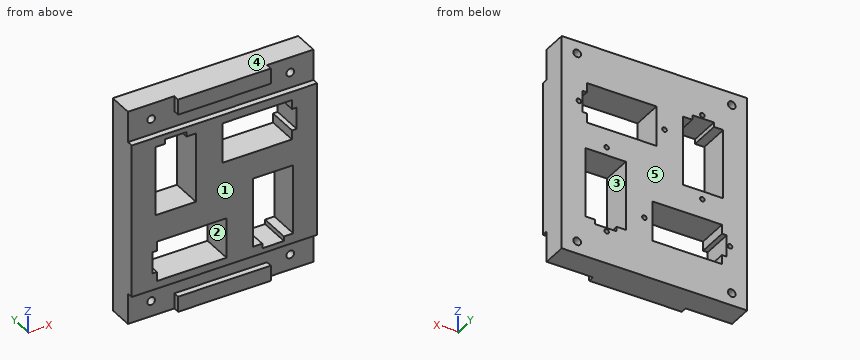
Autodesk Inventor part; units mm, degrees
ref_plane "YZ Plane" through (0, 0, 0) normal (1, 0, 0) x (0, 1, 0)
ref_plane "XZ Plane" through (0, 0, 0) normal (0, 1, 0) x (-1, 0, 0)
ref_plane "XY Plane" through (0, 0, 0) normal (0, 0, 1) x (1, 0, 0)
sketch "Skizze1" plane through (0, 0, 0) normal (0, 1, 0) x (-1, 0, 0)
  line L0 (30, -35) -> (-30, -35)
  line L1 (-30, -35) -> (-30, 35)
  line L2 (-30, 35) -> (30, 35)
  line L3 (30, 35) -> (30, -35)
  line L4 (30, -35) -> (-30, 35) construction
  line L5 (-30, -35) -> (30, 35) construction
  point P0 (0, 0)
  dimension "d0" = 60
  dimension "d1" = 70
extrude "Extrusion1" add sketch "Skizze1" along normal blind 10
sketch "Skizze2" plane through (0, 10, 0) normal (0, 1, 0) x (1, 0, 0)
  circle A0 centre (-15.75, 15.75) radius 1.75
  circle A1 centre (15.75, 15.75) radius 1.75
  circle A2 centre (15.75, -15.75) radius 1.75
  circle A3 centre (-15.75, -15.75) radius 1.75
  line L0 (42, 0) -> (-42, 0)
  line L1 (0, 49) -> (0, -49)
  point P0 (0, 0)
  dimension "d4" = 31.5
  dimension "d5" = 31.5
  dimension "d6" = 15.75
  dimension "d7" = 31.5
  dimension "d8" = 31.5
  dimension "d9" = 15.75
  dimension "d10" = 15.75
  dimension "d11" = 15.75
  dimension "d12" = 3.5
  dimension "d13" = 3.5
  dimension "d14" = 3.5
  dimension "d15" = 3.5
extrude "Extrusion2" cut sketch "Skizze2" against normal blind 10
sketch "Skizze3" plane through (0, 10, 0) normal (0, 1, 0) x (1, 0, 0)
  circle A0 centre (-15.75, 15.75) radius 1.75
  circle A1 centre (-15.75, 15.75) radius 5
  circle A2 centre (15.75, 15.75) radius 1.75
  circle A3 centre (15.75, 15.75) radius 5
  circle A4 centre (15.75, -15.75) radius 1.75
  circle A5 centre (15.75, -15.75) radius 5
  circle A6 centre (-15.75, -15.75) radius 1.75
  circle A7 centre (-15.75, -15.75) radius 5
  point P0 (0, 0)
  dimension "d18" = 10
  dimension "d19" = 10
  dimension "d20" = 10
  dimension "d21" = 10
extrude "Extrusion3" cut sketch "Skizze3" against normal blind 7 contours A0 | A1 | A2 | A3 | A4 | A5 | A6 | A7
sketch "Skizze6" plane through (0, 0, 0) normal (0, 1, 0) x (-1, 0, 0)
  line L0 (37.5, 25) -> (-37.5, 25)
  line L1 (37.5, -25) -> (-37.5, -25)
  line L2 (37.5, 40) -> (15, 40)
  line L3 (15, 40) -> (15, 30)
  line L4 (-37.5, 40) -> (-15, 40)
  line L5 (-15, 40) -> (-15, 30)
  line L6 (0, -45.47) -> (0, 45.495)
  line L7 (37.5, -40) -> (15, -40)
  line L8 (15, -40) -> (15, -30)
  line L9 (-37.5, -40) -> (-15, -40)
  line L10 (-15, -40) -> (-15, -30)
  line L11 (-15, 30) -> (15, 30)
  line L12 (-15, -30) -> (15, -30)
  line L13 (-37.5, 25) -> (-37.5, 40)
  line L14 (37.5, 40) -> (37.5, 25)
  line L15 (-37.5, -25) -> (-37.5, -40)
  line L16 (-30, 35) -> (-30, -35)
  line L17 (37.5, -25) -> (37.5, -40)
  point P0 (0, 0)
  dimension "d37" = 10
  dimension "d38" = 15
  dimension "d39" = 15
  dimension "d40" = 75
  dimension "d43" = 10
  dimension "d44" = 15
  dimension "d45" = 15
  dimension "d46" = 22.5
  dimension "d47" = 22.5
  dimension "d48" = 22.5
  dimension "d49" = 75
  dimension "d50" = 22.5
  dimension "d76" = 5
  dimension "d77" = 25
  dimension "d78" = 5
  dimension "d79" = 25
extrude "Extrusion6" cut sketch "Skizze6" along normal blind 2 contours L0 L6 L11 L3 L2 L14 | L0 L13 L4 L5 L11 L6 | L6 L12 L10 L9 L15 L1 | L1 L17 L7 L8 L12 L6
sketch "Skizze7" plane through (0, 2, 0) normal (0, -1, 0) x (1, 0, 0)
  circle A0 centre (-22.5, 30) radius 1.25
  circle A1 centre (22.5, 30) radius 1.25
  circle A2 centre (22.5, -30) radius 1.25
  circle A3 centre (-22.5, -30) radius 1.25
  line L0 (0, 49) -> (0, -49)
  line L1 (-42, 0) -> (42, 0)
  point P0 (0, 0)
  dimension "d55" = 45
  dimension "d56" = 22.5
  dimension "d57" = 60
  dimension "d58" = 45
  dimension "d59" = 60
  dimension "d60" = 30
  dimension "d61" = 30
  dimension "d62" = 2.5
  dimension "d63" = 2.5
  dimension "d64" = 2.5
  dimension "d65" = 2.5
  dimension "d71" = 22.5
extrude "Extrusion7" cut sketch "Skizze7" against normal blind 6
sketch "Skizze9" plane through (0, 10, 0) normal (0, 1, 0) x (1, 0, 0)
  line L0 (-9.25, -21.85) -> (-22.25, -21.85)
  line L1 (-22.25, -21.85) -> (-22.25, 0.65)
  line L2 (-22.25, 0.65) -> (-9.25, 0.65)
  line L3 (-9.25, 0.65) -> (-9.25, -21.85)
  circle A0 centre (-15.75, -15.75) radius 1.75
  line L4 (21.85, -22.25) -> (-0.65, -22.25)
  line L5 (-0.65, -22.25) -> (-0.65, -9.25)
  line L6 (-0.65, -9.25) -> (21.85, -9.25)
  line L7 (21.85, -9.25) -> (21.85, -22.25)
  line L8 (22.25, 21.85) -> (9.25, 21.85)
  line L9 (9.25, 21.85) -> (9.25, -0.65)
  line L10 (9.25, -0.65) -> (22.25, -0.65)
  line L11 (22.25, -0.65) -> (22.25, 21.85)
  circle A1 centre (15.75, 15.75) radius 1.75
  line L12 (-21.85, 9.5) -> (0.65, 9.5)
  line L13 (0.65, 9.5) -> (0.65, 22.5)
  line L14 (0.65, 22.5) -> (-21.85, 22.5)
  line L15 (-21.85, 22.5) -> (-21.85, 9.5)
  circle A2 centre (15.75, -15.75) radius 1.75
  point P0 (0, 0)
  point P1 (-15.75, 16)
  dimension "d80" = 13
  dimension "d81" = 22.5
  dimension "d82" = 6.5
  dimension "d83" = 6.1
  dimension "d97" = 13
  dimension "d99" = 22.5
  dimension "d101" = 13
  dimension "d102" = 6.5
  dimension "d103" = 6.1
  dimension "d104" = 22.5
  dimension "d105" = 13
  dimension "d106" = 22.5
  dimension "d107" = 6.1
  dimension "d108" = 6.5
  dimension "d164" = 6.5
extrude "Extrusion9" cut sketch "Skizze9" against normal blind 10 contours L0 L1 L2 L3 | L4 L5 L6 L7 | L11 L10 L9 L8 | A1 | L15 L14 L13 L12 | A2
sketch "Skizze10" plane through (0, 10, 0) normal (0, 1, 0) x (1, 0, 0)
  circle A0 centre (-3.25, -15.5) radius 0.75
  circle A1 centre (24.45, -15.5) radius 0.75
  circle A2 centre (15.5, -3.25) radius 0.75
  circle A3 centre (15.5, 24.45) radius 0.75
  circle A4 centre (3.25, 15.75) radius 0.75
  circle A5 centre (-24.45, 15.75) radius 0.75
  circle A6 centre (-15.5, 3.25) radius 0.75
  circle A7 centre (-15.5, -24.45) radius 0.75
  line L0 (-22.25, 0.65) -> (-9.25, 0.65)
  line L1 (-9.25, -21.85) -> (-22.25, -21.85)
  line L2 (-21.85, 9.5) -> (-21.85, 22.5)
  line L3 (0.65, 22.5) -> (0.65, 9.5)
  line L4 (9.25, 21.85) -> (22.25, 21.85)
  line L5 (22.25, -0.65) -> (9.25, -0.65)
  line L6 (21.85, -9.25) -> (21.85, -22.25)
  line L7 (-0.65, -22.25) -> (-0.65, -9.25)
  line L8 (-9.25, 0.65) -> (-9.25, -21.85)
  line L9 (-0.65, -9.25) -> (21.85, -9.25)
  line L10 (9.25, -0.65) -> (9.25, 21.85)
  line L11 (0.65, 9.5) -> (-21.85, 9.5)
  point P0 (0, 0)
  dimension "d109" = 1.5
  dimension "d110" = 1.5
  dimension "d111" = 1.5
  dimension "d112" = 1.5
  dimension "d113" = 1.5
  dimension "d114" = 1.5
  dimension "d115" = 1.5
  dimension "d116" = 1.5
  dimension "d117" = 2.6
  dimension "d118" = 2.6
  dimension "d119" = 2.6
  dimension "d120" = 2.6
  dimension "d121" = 2.6
  dimension "d122" = 2.6
  dimension "d123" = 2.6
  dimension "d124" = 2.6
  dimension "d125" = 6.25
  dimension "d126" = 6.25
  dimension "d127" = 6.25
  dimension "d128" = 6.25
  dimension "d130" = 6.25
  dimension "d131" = 6.25
  dimension "d132" = 6.25
  dimension "d133" = 6.25
extrude "Extrusion10" cut sketch "Skizze10" against normal blind 5
sketch "Skizze11" plane through (0, 10, 0) normal (0, 1, 0) x (1, 0, 0)
  circle A0 centre (25, -31) radius 1.25
  circle A1 centre (-25, -31) radius 1.25
  circle A2 centre (-25, 31) radius 1.25
  circle A3 centre (25, 31) radius 1.25
  line L0 (-30, -35) -> (30, -35)
  line L1 (30, -35) -> (30, 35)
  point P0 (0, 0)
  dimension "d136" = 50
  dimension "d137" = 62
  dimension "d138" = 50
  dimension "d139" = 62
  dimension "d140" = 4
  dimension "d141" = 5
  dimension "d142" = 5
  dimension "d143" = 4
  dimension "d144" = 2.5
  dimension "d145" = 2.5
  dimension "d146" = 2.5
  dimension "d147" = 2.5
extrude "Extrusion11" cut sketch "Skizze11" against normal blind 5
sketch "Skizze12" plane through (0, 10, 0) normal (0, 1, 0) x (1, 0, 0)
  line L0 (-21.85, 22.5) -> (-21.85, 9.5)
  line L1 (-21.85, 12.5) -> (-23.35, 12.5)
  line L2 (-23.35, 12.5) -> (-23.35, 19.5)
  line L3 (-23.35, 19.5) -> (-21.85, 19.5)
  line L4 (-21.85, 19.5) -> (-21.85, 12.5)
  line L5 (9.25, 21.85) -> (22.25, 21.85)
  line L6 (19.25, 21.85) -> (12.25, 21.85)
  line L7 (12.25, 21.85) -> (12.25, 23.35)
  line L8 (12.25, 23.35) -> (19.25, 23.35)
  line L9 (19.25, 23.35) -> (19.25, 21.85)
  line L10 (21.85, -9.25) -> (21.85, -22.25)
  line L11 (21.85, -19.25) -> (23.35, -19.25)
  line L12 (23.35, -19.25) -> (23.35, -12.25)
  line L13 (23.35, -12.25) -> (21.85, -12.25)
  line L14 (21.85, -12.25) -> (21.85, -19.25)
  line L15 (-9.25, -21.85) -> (-22.25, -21.85)
  line L16 (-12.25, -21.85) -> (-19.25, -21.85)
  line L17 (-19.25, -21.85) -> (-19.25, -23.35)
  line L18 (-19.25, -23.35) -> (-12.25, -23.35)
  line L19 (-12.25, -23.35) -> (-12.25, -21.85)
  line L20 (21.85, -22.25) -> (-0.65, -22.25)
  line L21 (-0.65, -9.25) -> (21.85, -9.25)
  line L22 (-9.25, 0.65) -> (-9.25, -21.85)
  line L23 (-22.25, -21.85) -> (-22.25, 0.65)
  line L24 (-21.85, 22.5) -> (0.65, 22.5)
  line L25 (0.65, 9.5) -> (-21.85, 9.5)
  line L26 (9.25, -0.65) -> (9.25, 21.85)
  line L27 (22.25, 21.85) -> (22.25, -0.65)
  point P0 (0, 0)
  point P1 (-21.85, 19.5)
  dimension "d150" = 3
  dimension "d151" = 3
  dimension "d152" = 1.5
  dimension "d153" = 3
  dimension "d154" = 3
  dimension "d155" = 1.5
  dimension "d156" = 3
  dimension "d157" = 3
  dimension "d158" = 1.5
  dimension "d159" = 3
  dimension "d160" = 3
  dimension "d161" = 1.5
extrude "Extrusion12" cut sketch "Skizze12" against normal blind 10
equation "\"d6\" = 0.5 * d5"
equation "\"d9\" = 0.5 * d7"
equation "\"d10\" = 0.5 * d8"
equation "\"d11\" = 0.5 * d5"
equation "\"d56\" = 0.5 * d55"
equation "\"d60\" = 0.5 * d57"
equation "\"d61\" = 0.5 * d59"
equation "\"d71\" = 0.5 * d58"
equation "\"d82\" = 0.5 * d80"
equation "\"d102\" = 0.5 * d101"
equation "\"d164\" = 0.5 * d97"
properties part number "Fuehrungsgrundplatte_V2"
CAD build for the part. Positions are in the model's coordinates, mm. Face numbers are marked on the shaded views. A direction names the side the tool comes from. Coordinates: 2 decimals unless noted, no trailing zeros. Write each loop counter-clockwise with the first axis right and the second up, starting at its lowest first coordinate (ties: lowest second). Pieces come first, ordered by that corner, then holes. Notation, with made-up numbers: (-17.5, 16) -> (-7.5, 16) arc R24 cw to (-7.5, 51) -> close; hole circle Ø11 at (62, 14.25). An arc over 180 degrees is marked (long way). Use CSV: the item, a comma, the result in double quotes. Start each with the question number.
Item 1: Band-saw the part on D-D, the plane z = -7. Write the cut outline in (x, y).
Item 2: Wall check: probe 1 along X at (y, z) = (6.9, 15.5); probe 2 along Z at (x, y) = (15.5, 7.4); probe 3 along Z at (x, y) = (-11, 3.5). Give the ranges that are in metal, low to high.
Item 3: Band-saw the part on C-C, the plane y = 1.25. Give the number of separate pieces and of enclosed holes in the cut face, plus the area to 3 significant figures.
Item 4: Drop flat-ended pins along their axis: P1, Ø2, axis at x = 25, z = 31, coming from the +Y side; P2, Ø0.9, axis at x = 15.5, z = -24.45, coming from the -Y side; P3, Ø4, axis at x = -25, z = 31, coming from the -Y side; P4, Ø1, axis at y = 1, z = -32.5, coming from the +X side. Give the stop position or say it passes through.
Item 5: Band-saw the part on B-B, the plane x = -6. Write the cut outline in (y, z).
Item 6: Band-saw the part on A-A, the plane x = -20. Write the cut outline in (y, z).
Item 7: Tool access for the marked faces 1 and 2: list every direction of +Z, -Z, +X, -X, +Y, -Y with a clear straight run to the whole face (end or side of a thin tool).
Item 8: Two-plate mould, pull along Z, no slides. Class the marked faces 3, 4 and 5: +Z half, -Z half, draft (parallel to the pull), parting line (faces both ways), or undercut.
Response values:
1,outline,"(-30, 0) -> (9.25, 0) -> (9.25, 10) -> (-30, 10) -> close; (22.25, 0) -> (30, 0) -> (30, 10) -> (22.25, 10) -> close"
2,probe 1,"x = -30 to -22.25, -9.25 to -4, -2.5 to -0.65, 23.35 to 23.7, 25.2 to 30"
2,probe 2,"z = -35 to -25.2, -23.7 to -23.35, 0.65 to 2.5, 4 to 9.25, 22.25 to 35"
2,probe 3,"z = -35 to -22.5, -9.5 to -0.65, 21.85 to 35"
3,separate pieces,"3"
3,enclosed holes,"4"
3,area,"2,090 mm2"
4,P1,"stops at y = 5"
4,P2,"stops at y = 0"
4,P3,"stops at y = 2"
4,P4,"stops at x = 15"
5,outline,"(0, -35) -> (10, -35) -> (10, -22.5) -> (0, -22.5) -> (0, -25) -> (2, -25) -> (2, -30) -> (0, -30) -> close; (0, -9.5) -> (10, -9.5) -> (10, 35) -> (0, 35) -> (0, 30) -> (2, 30) -> (2, 25) -> (0, 25) -> close"
6,outline,"(0, -25) -> (2, -25) -> (2, -35) -> (10, -35) -> (10, -22.5) -> (0, -22.5) -> close; (0, -9.5) -> (10, -9.5) -> (10, -0.65) -> (0, -0.65) -> close; (0, 21.85) -> (10, 21.85) -> (10, 35) -> (2, 35) -> (2, 25) -> (0, 25) -> close"
7,face 1,"+Z, -Z, +X, -X, -Y"
7,face 2,"+Y, -Y"
8,face 3,"undercut"
8,face 4,"+Z half"
8,face 5,"draft"
